Geometry check sheet. Reference: the model listing, model coordinates, mm. A direction names the side the tool comes from. Coordinates: 2 decimals unless noted, no trailing zeros. Loops run counter-clockwise (first coordinate to the right, second up) from the corner with the lowest first, then second, coordinate; pieces in that order, holes last. Notation, with made-up numbers: M -13.5,77 L 29.5,77 A21 ccw 29.5,90 Z; hole C 11.25,69 d3. An arc over 180 degrees is marked long. One line per question, with ' | ' between items. Start each with the question number.
Autodesk Inventor part; units mm, degrees
ref_plane "Work Plane1" through (0, 66.3321, 0) normal (0, -1, 0) x (1, 0, 0)
ref_plane "YZ Plane" through (0, 0, 0) normal (1, 0, 0) x (0, 1, 0)
ref_plane "XZ Plane" through (0, 0, 0) normal (0, 1, 0) x (-1, 0, 0)
sketch "Sketch1" plane through (0, 0, 0) normal (0, 0, 1) x (1, 0, 0)
  line L0 (0, 0) -> (233.68, 0)
  line L1 (233.68, 0) -> (233.68, 132.6642)
  line L2 (233.68, 132.6642) -> (0, 132.6642)
  line L3 (0, 132.6642) -> (0, 0)
  dimension "d0" = 132.6642
  dimension "d1" = 233.68
extrude "Extrusion1" add sketch "Sketch1" along normal blind 29.21
sketch "Sketch2" plane through (0, 0, 29.21) normal (0, 0, 1) x (1, 0, 0)
  line L0 (-0.3825, 3.8354) -> (233.706, 3.8354)
  line L1 (233.706, 3.8354) -> (233.706, 128.8288)
  line L2 (233.706, 128.8288) -> (-0.3825, 128.8288)
  line L3 (-0.3825, 128.8288) -> (-0.3825, 3.8354)
  line L4 (233.68, 132.6642) -> (0, 132.6642)
  line L5 (0, 0) -> (233.68, 0)
  dimension "d4" = 3.8354
  dimension "d5" = 3.8354
extrude "Extrusion2" cut sketch "Sketch2" against normal blind 21.4884
sketch "Sketch3" plane through (0, 0, 29.21) normal (0, 0, 1) x (1, 0, 0)
  line L0 (233.68, 0) -> (119.38, 0)
  line L1 (119.38, 0) -> (119.38, 3.8354)
  line L2 (119.38, 3.8354) -> (233.68, 3.8354)
  line L3 (233.68, 3.8354) -> (233.68, 0)
  point P0 (0, 0)
  dimension "d8" = 114.3
  dimension "d9" = 3.8354
extrude "Extrusion3" cut sketch "Sketch3" against normal blind 21.4884
sketch "Sketch4" plane through (0, 0, 0) normal (0, 0, -1) x (-1, 0, 0)
  line L0 (-233.68, 0) -> (-233.68, 132.6642)
  line L1 (-233.68, 132.6642) -> (-203.2, 132.6642)
  line L2 (-203.2, 132.6642) -> (-203.2, 128.8288)
  line L3 (-203.2, 128.8288) -> (-233.68, 128.8288)
  line L4 (-233.68, 128.8288) -> (-233.68, 132.6642)
  line L5 (-233.68, 0) -> (-203.2, 0)
  line L6 (-203.2, 0) -> (-203.2, 3.8354)
  line L7 (-203.2, 3.8354) -> (-233.68, 3.8354)
  line L8 (-233.68, 3.8354) -> (-233.68, 0)
  point P0 (0, 0)
  dimension "d12" = 3.8354
  dimension "d13" = 30.48
  dimension "d14" = 3.8354
  dimension "d15" = 30.48
extrude "Extrusion4" add sketch "Sketch4" along normal blind 31.75
sketch "Sketch7" plane through (0, 132.6642, 29.21) normal (0, 1, 0) x (1, 0, 0)
  circle A0 centre (217.8629, 48.5394) radius 2.54
  circle A1 centre (217.8134, 38.7605) radius 1.3589
  circle A2 centre (224.7426, 41.5897) radius 1.3589
  circle A3 centre (227.6418, 48.4899) radius 1.3589
  circle A4 centre (224.8126, 55.4191) radius 1.3589
  circle A5 centre (217.9124, 58.3182) radius 1.3589
  circle A6 centre (210.9832, 55.4891) radius 1.3589
  circle A7 centre (208.084, 48.5889) radius 1.3589
  circle A8 centre (210.9132, 41.6597) radius 1.3589
  point P0 (0, 29.21)
  dimension "d39" = 5.08
  dimension "d40" = 2.7178
  dimension "d41" = 9.779
  dimension "d44" = 360
extrude "Extrusion7" cut sketch "Sketch7" against normal blind 12.7 contours A1 | A2 | A3 | A4 | A5 | A6 | A7 | A8
ref_plane "Work Plane1" through (0, 66.3321, 0) normal (0, -1, 0) x (1, 0, 0)
mirror "Mirror2" about plane through (0, 66.3321, 0) normal (0, -1, 0) of "Extrusion7"
sketch "Sketch9" plane through (0, 0, 0) normal (0, -1, 0) x (1, 0, 0)
  circle A0 centre (157.48, 2.6482) radius 1.3589
  circle A1 centre (176.9362, 2.7347) radius 1.3589
  line L0 (119.38, 7.7216) -> (119.38, 29.21)
  point P0 (0, 0)
  dimension "d57" = 2.7178
  dimension "d58" = 19.4564
  dimension "d59" = 2.7178
  dimension "d60" = 38.1
extrude "Extrusion9" cut sketch "Sketch9" against normal blind 12.7
properties part number "Guide"
1. Sectioned sample at A-A (z = 17). Record the cut outline in (x, y).
2. Tool access check on faces 1 (the flat face through (118, 128.829, 19)), 2 (the flat face through (218, 128.829, -16)), 3 (the flat face through (118, 132.664, 12)). Record the directions out of +Z, -Z, +X, -X, +Y, -Y that give a thin tool (end or side, any length) a straight path to the whole face; none if there is none.
3. Sectioned sample at B-B (y = 35.5). Record the cut outline in (x, z), and give its area (3 significant figures).
4. Thickness scan on line 1 (Y direction, x = 33.5, z = 8.5); line 2 (Y direction, x = 186, z = 13); line 3 (Z direction, x = 95, y = 75). Record the ranges inside material, lowest first.
5. Depth check by flat-ended pin: pin 1 Ø1.6 at (x, z) = (217.81, -9.55) entering from -Y; pin 2 Ø1.4 at (x, z) = (157.5, 3) entering from -Y; pin 3 Ø3 at (y, z) = (1, 23) entering from +X; pin 4 Ø3 at (y, z) = (1.5, -13.5) entering from -X. Enter the tip coordinate at first touch or a pass-through.
Result:
1) outline: M 0,0 L 119.38,0 L 119.38,3.84 L 0,3.84 Z; M 0,128.83 L 233.68,128.83 L 233.68,132.66 L 0,132.66 Z
2) face 1: +Z, +X, -X | face 2: -Z, +X, -X | face 3: +Z, -Z, +X, -X, +Y
3) outline: M 0,0 L 233.68,0 L 233.68,7.72 L 0,7.72 Z | area: 1,800 mm2
4) line 1: y = 0 to 3.84, 128.83 to 132.66 | line 2: y = 128.83 to 132.66 | line 3: z = 0 to 7.72
5) pin 1: passes through | pin 2: stops at y = 12.7 | pin 3: stops at x = 119.38 | pin 4: stops at x = 203.2
